Design review of the part shown in the three views and the two pictorial views. Dimensions are in mm from the part's minimum x, y and z. Coordinates: 2 decimals unless noted, no trailing zeros. Loops run counter-clockwise (first coordinate to the right, second up) from the corner with the lowest first, then second, coordinate; pieces in that order, holes last. Notation, with made-up numbers: (87, 57) -> (107, 57) arc R19 cw to (107, 79) -> close; hole circle Ø7 at (54, 28). An arc over 180 degrees is marked (long way). One line per item, written item: value. Start each with the question number.
1. Add section D-D on y = 37. Write out the cut boundary in (x, z).
2. Add section B-B on z = 124.5. Write out the cut boundary in (x, y), plus the area to 3 significant figures.
3. Insertion check: pin 1 (7 mm diameter, centred on x = 11, y = 2, fed in from -Z); pin 2 (3 mm diameter, centred on y = 2, z = 109.5, fed in from -X). Each pin has a flat end and moves straight along its axis. Give the tip position at first contact, or say it passes through.
4. For probe 1 along Z at (x, y) = (9, 38.5); probe 2 along Y at (x, z) = (1.5, 102); probe 3 along X at (y, z) = (18.5, 10), list the stretches that pass through material, from the lowest coordinate up.
5. Add section A-A on x = 10.75. Write out the cut boundary in (y, z).
6. Draft analysis for pull direction Z (two halves, no side actions). For the marked faces 1, 2, 3 and 4, state which applies: pulls with the +Z half, pulls with the -Z half, needs draft (parallel to the pull), parting line crosses it, or undercut.
7. Add section C-C on x = 17.25. Write out the cut boundary in (y, z), plus the area to 3 significant figures.
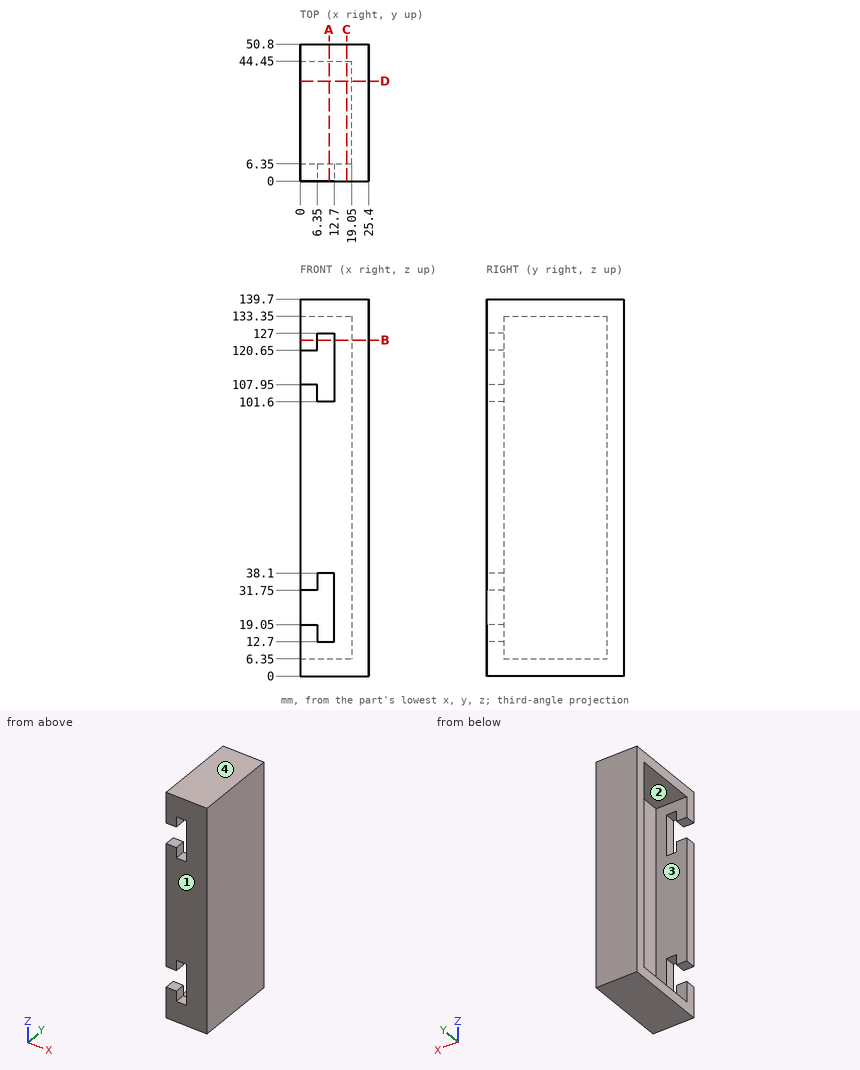
Worked answers:
1. outline: (0, 0) -> (25.4, 0) -> (25.4, 139.7) -> (0, 139.7) -> (0, 133.35) -> (19.05, 133.35) -> (19.05, 6.35) -> (0, 6.35) -> close
2. outline: (0, 0) -> (6.35, 0) -> (6.35, 6.35) -> (0, 6.35) -> close; (0, 44.45) -> (19.05, 44.45) -> (19.05, 6.35) -> (12.7, 6.35) -> (12.7, 0) -> (25.4, 0) -> (25.4, 50.8) -> (0, 50.8) -> close
2. area: 524 mm²
3. pin 1: stops at z = 0
3. pin 2: stops at x = 12.7
4. probe 1: z = 0 to 6.35, 133.35 to 139.7
4. probe 2: y = 0 to 6.35, 44.45 to 50.8
4. probe 3: x = 19.05 to 25.4
5. outline: (0, 0) -> (50.8, 0) -> (50.8, 139.7) -> (0, 139.7) -> (0, 127) -> (6.35, 127) -> (6.35, 133.35) -> (44.45, 133.35) -> (44.45, 6.35) -> (6.35, 6.35) -> (6.35, 12.7) -> (0, 12.7) -> close; (0, 38.1) -> (6.35, 38.1) -> (6.35, 101.6) -> (0, 101.6) -> close
6. face 1: needs draft
6. face 2: undercut
6. face 3: undercut
6. face 4: pulls with the +Z half
7. outline: (0, 0) -> (50.8, 0) -> (50.8, 139.7) -> (0, 139.7) -> close; hole (6.35, 6.35) -> (44.45, 6.35) -> (44.45, 133.35) -> (6.35, 133.35) -> close
7. area: 2,260 mm²
